Verification items for the finished model (mm, model axes). A direction names the side the tool comes from. Coordinates: 2 decimals unless noted, no trailing zeros. Order: outer loops, then holes, each group sorted by start corner. A loop starts at its lowest first (then second) coordinate and runs counter-clockwise, first axis right, second up. Notation, with made-up numbers: M -16.75,-1.5 L 22.25,-1.5 A11 ccw 22.25,12.5 Z; hole C -36.75,43.25 d1. An arc over 180 degrees is marked long. Return JSON: item names as keys, results as strings. Group by question number.
1. Mould release check, pull along X, two halves, no side actions. Record for faces 1 (the cylindrical face through (0.91, 2.72, 80.16)), 2 (the cylindrical face through (0.94, 2.23, 9.65)), 3 (the flat face through (5, 2.4, 44)), 4 (the flat face through (3, 1, 86)): +X half, -X half, draft (parallel to the pull), parting line (faces both ways), or undercut.
2. Set-up check for faces 5 (the flat face through (7, 3, 44)), 6 (the flat face through (3, 1, 45)): record each of +Z, -Z, +X, -X, +Y, -Y from which the full face is reachable in a straight line by a thin tool's end or side.
3. Section check D-D, the plane z = 64. Record the cut outline in (x, y).
4. Section check C-C, the plane x = 5.75. Record the cut outline in (y, z).
5. Material ranges on line 1 along Z through (x, y) = (2, 2.9); line 2 along Z through (x, y) = (2.5, 2.05); line 3 along X through (y, z) = (2.85, 80), recorded low to high.
6. Section check A-A, the plane z = 80. Record the cut outline in (x, y).
7. Gauge pin test, flat ends, axial feed: pin 1 (1.9 mm diameter, centred on y = 1, z = 85.5, fed in from +X); pin 2 (1.2 mm diameter, centred on x = 6, z = 32, fed in from -Y); pin 3 (3 mm diameter, centred on x = 2.5, z = 80, fed in from +Y). Record the tip position at first contact, or that the pin passes through.
8. Section check B-B, the plane y = 1.1. Record the cut outline in (x, z).
```python
from build123d import *

# Parameters (mm, degrees)
EXTRUDE_1_DEPTH     = 90
SKETCH_2_R          = 1.6
CUT_EXTRUDE_1_DEPTH = 91.378979857


with BuildPart() as part:
    # 草图1 → 凸台-拉伸1 (new body)
    with BuildSketch(Plane.XY):
        Polygon((3, 0), (3, 2.4), (7, 2.4), (7, 4.4), (0, 4.4), (0, 0), align=None)
    extrude(amount=EXTRUDE_1_DEPTH)

    # 草图2 → 切除-拉伸1 (cut, through all)
    with BuildSketch(Plane(origin=(0, 4.4, 0), x_dir=(1, 0, 0), z_dir=(0, 1, 0))):
        with Locations(Location((2.5, -37, 0), (0, 0, 270))):
            Circle(SKETCH_2_R)
        with Locations(Location((2.5, -10, 0), (0, 0, 270))):
            Circle(SKETCH_2_R)
        with Locations(Location((2.5, -80, 0), (0, 0, 288.209956864))):
            Circle(SKETCH_2_R)
        with Locations(Location((2.5, -53, 0), (0, 0, 288.209956864))):
            Circle(SKETCH_2_R)
    extrude(amount=-CUT_EXTRUDE_1_DEPTH, mode=Mode.SUBTRACT)


solid = part.part
```
Answers follow:
{
 "1": {"face 1": "undercut", "face 2": "undercut", "face 3": "draft", "face 4": "+X half"},
 "2": {"face 5": "+Z, -Z, +X, +Y, -Y", "face 6": "+Z, -Z, +X, -Y"},
 "3": {"outline": "M 0,0 L 3,0 L 3,2.4 L 7,2.4 L 7,4.4 L 0,4.4 Z"},
 "4": {"outline": "M 2.4,0 L 4.4,0 L 4.4,90 L 2.4,90 Z"},
 "5": {"line 1": "0 to 8.48, 11.52 to 35.48, 38.52 to 51.48, 54.52 to 78.48, 81.52 to 90", "line 2": "0 to 8.4, 11.6 to 35.4, 38.6 to 51.4, 54.6 to 78.4, 81.6 to 90", "line 3": "0 to 0.9, 4.1 to 7"},
 "6": {"outline": "M 0,0 L 0.9,0 L 0.9,4.4 L 0,4.4 Z; M 4.1,2.4 L 7,2.4 L 7,4.4 L 4.1,4.4 Z"},
 "7": {"pin 1": "x = 3", "pin 2": "y = 2.4", "pin 3": "through"},
 "8": {"outline": "M 0,0 L 3,0 L 3,8.48 A1.6 cw long 3,11.52 L 3,35.48 A1.6 cw long 3,38.52 L 3,51.48 A1.6 cw long 3,54.52 L 3,78.48 A1.6 cw long 3,81.52 L 3,90 L 0,90 Z"}
}
